Input: dimensioned drawing with shaded views. Units: mm. Origin: part minimum x, y, z. A direction names the side the tool comes from. Give positions to 0.01 mm unless a question says otherwise; leave off trailing zeros. Order: outer loops, then holes, each group sorted by start corner. A loop starts at its lowest first (then second) coordinate and runs counter-clockwise, first axis right, second up. Notation, with made-up numbers: (14.25, 71.25) -> (34.25, 71.25) arc R35 cw to (34.25, 104.25) -> close; hole circle Ø5 at (17, -8). An arc over 180 degrees is marked (long way). Use CSV: the item, a comma, the result in double quotes.
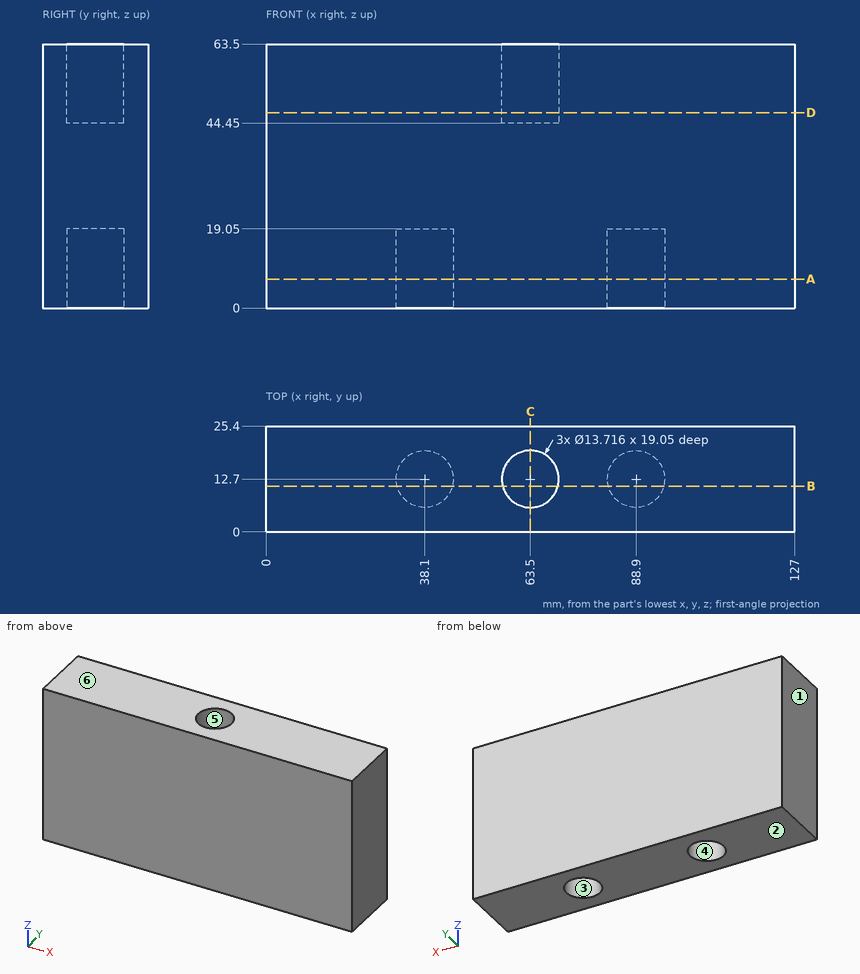
1. Ray query, line 1 along Y through (x, z) = (63, 48); line 2 along Y through (x, z) = (38.1, 12); line 3 along X through (y, z) = (15.75, 14). Return the intervals inside material, ascending.
Answer below:
line 1,"y = 0 to 5.86, 19.54 to 25.4"
line 2,"y = 0 to 5.84, 19.56 to 25.4"
line 3,"x = 0 to 31.96, 44.24 to 82.76, 95.04 to 127"
2. Pin query (flat end, axial travel): P1, Ø11, axis at x = 88.9, y = 12.7, coming from the -Z side; P2, Ø11, axis at x = 63.5, y = 12.7, coming from the +Z side. Return the tip coordinate at first contact, or that it passes through.
Answer below:
P1,"stops at z = 19.05"
P2,"stops at z = 44.45"
3. Section query B-B on y = 11. Return loops of the section in (x, z), plus the area to 3 significant figures.
Answer below:
outline,"(0, 0) -> (31.46, 0) -> (31.46, 19.05) -> (44.74, 19.05) -> (44.74, 0) -> (82.26, 0) -> (82.26, 19.05) -> (95.54, 19.05) -> (95.54, 0) -> (127, 0) -> (127, 63.5) -> (70.14, 63.5) -> (70.14, 44.45) -> (56.86, 44.45) -> (56.86, 63.5) -> (0, 63.5) -> close"
area,"7,310 mm²"
4. Access query for the marked faces 4, 5 and 6. Directions: +Z, -Z, +X, -X, +Y, -Y. A direction counts if a zero-diameter tool reaches every point of the face in a straight line with its end or side. Return the directions, or none.
Answer below:
face 4,"-Z"
face 5,"+Z"
face 6,"+Z, +X, -X, +Y, -Y"
5. Section query D-D on z = 47. Return loops of the section in (x, y).
Answer below:
outline,"(0, 0) -> (127, 0) -> (127, 25.4) -> (0, 25.4) -> close; hole circle Ø13.72 at (63.5, 12.7)"
6. Mould query, pull axis X, two halves, no side actions, for the marked faces 1, 2 and 3. Classes: released by +X, released by -X, zero draft, split by the parting line, or undercut.
Answer below:
face 1,"released by -X"
face 2,"zero draft"
face 3,"undercut"
7. Section query A-A on z = 7. Return loops of the section in (x, y).
Answer below:
outline,"(0, 0) -> (127, 0) -> (127, 25.4) -> (0, 25.4) -> close; hole circle Ø13.72 at (38.1, 12.7); hole circle Ø13.72 at (88.9, 12.7)"
8. Section query C-C on x = 63.5. Return loops of the section in (y, z), plus the area to 3 significant figures.
Answer below:
outline,"(0, 0) -> (25.4, 0) -> (25.4, 63.5) -> (19.56, 63.5) -> (19.56, 44.45) -> (5.84, 44.45) -> (5.84, 63.5) -> (0, 63.5) -> close"
area,"1,350 mm²"
